Here's the drawing with two shaded views (mm, measured from the low corner). I have some questions. A direction names the side the tool comes from. Round coordinates to 2 decimals unless told otherwise and drop trailing zeros. Loops run counter-clockwise (first coordinate to the right, second up) from the corner with the lowest first, then second, coordinate; pieces in that order, holes last. Notation, with made-up numbers: (45.5, -24.75) -> (77.5, -24.75) arc R3 ccw to (77.5, -19.75) -> close; hole circle Ø2 at (-2, 6). An arc over 180 degrees is marked (long way). Write item = value, one per line.
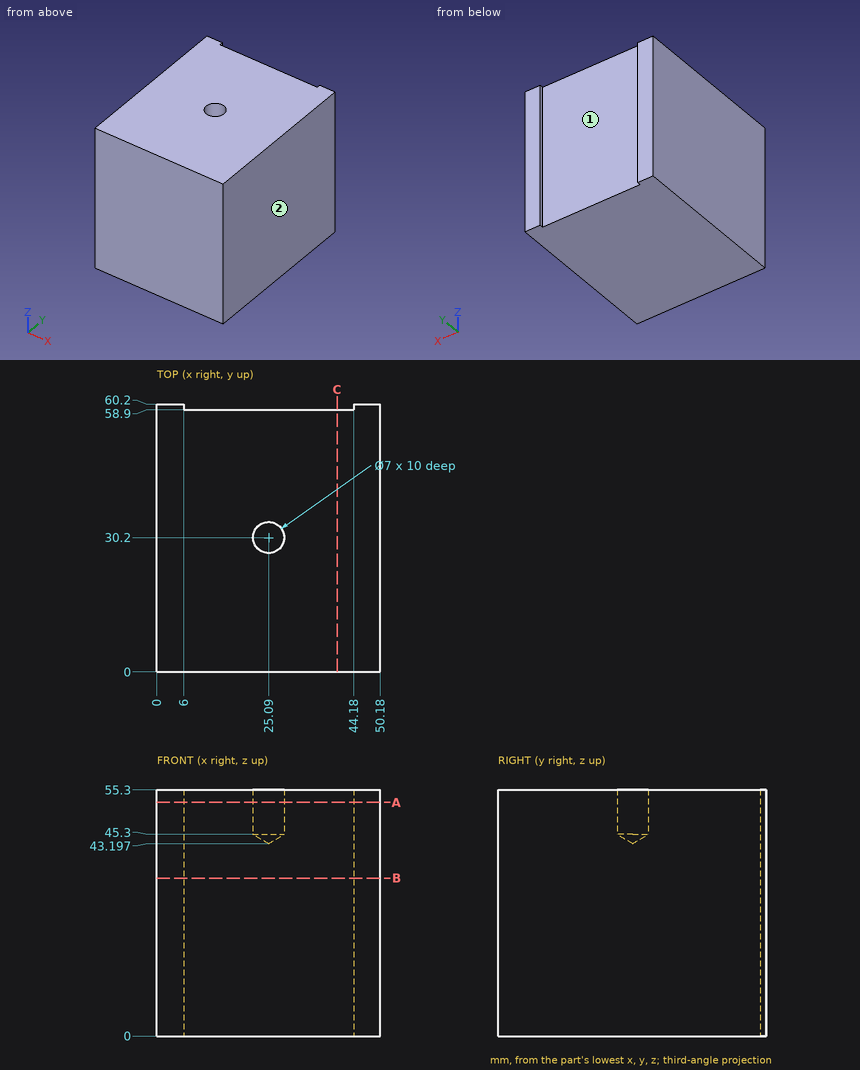
1. I need wall thicknesses on line 1 (Y direction, x = 25.09, z = 53); line 2 (X direction, y = 30, z = 47); line 3 (Y direction, x = 27, z = 22). Which ranges of each line are inside material? Lowest first, please. Write a range as [from, to].
Entries:
line_1 = [0, 26.7], [33.7, 58.9]
line_2 = [0, 21.6], [28.58, 50.18]
line_3 = [0, 58.9]
2. Suppose I cut it at A-A, the plane z = 52.5. List the corners of the cut face in (x, y) for me, and give its area (3 significant figures).
Entries:
outline = (0, 0) -> (50.18, 0) -> (50.18, 60.2) -> (44.18, 60.2) -> (44.18, 58.9) -> (6, 58.9) -> (6, 60.2) -> (0, 60.2) -> close; hole circle Ø7 at (25.09, 30.2)
area = 2,930 mm²
3. Suppose I cut it at C-C, the plane x = 40.5. List the corners of the cut face in (y, z) for me.
Entries:
outline = (0, 0) -> (58.9, 0) -> (58.9, 55.3) -> (0, 55.3) -> close
4. For the marked faces 1 and 2, which set-ups out of +Z, -Z, +X, -X, +Y, -Y let a thin tool reach every point of the face, with its end or its side?
Entries:
face_1 = +Z, -Z, +Y
face_2 = +Z, -Z, +X, +Y, -Y
5. I'm going to push flat-ended pins straight in: pin 1 (9 mm diameter, centred on x = 25.09, y = 30.2, fed in from -Z); pin 2 (8 mm diameter, centred on x = 17, z = 45.5, fed in from +Y). Where does each tip first touch, or does it pass through?
Entries:
pin_1 = 0
pin_2 = 58.9
6. Suppose I cut it at B-B, the plane z = 35.5. List the corners of the cut face in (x, y) for me, and give its area (3 significant figures).
Entries:
outline = (0, 0) -> (50.18, 0) -> (50.18, 60.2) -> (44.18, 60.2) -> (44.18, 58.9) -> (6, 58.9) -> (6, 60.2) -> (0, 60.2) -> close
area = 2,970 mm²
